Build history of the part. All positions in model axes, mm. Round coordinates to 2 decimals unless told otherwise and drop trailing zeros. Write each loop counter-clockwise with the first axis right and the second up, starting at its lowest first coordinate (ties: lowest second). Pieces come first, ordered by that corner, then holes.
Item 1: Band-saw the part on C-C, the plane z = 0. Write the cut outline in (x, y).
Item 2: Band-saw the part on A-A, the plane x = 29. Write the cut outline in (y, z), then the cut area to 3 significant figures.
Item 3: Wall check: probe 1 along X at (y, z) = (1.05, -0.5); probe 2 along X at (y, z) = (0.2, 3); probe 3 along X at (y, z) = (1.6, 0). Give the ranges that are in metal, low to high.
Item 4: Drop flat-ended pins along their axis: pin 1 Ø1.9 at (x, z) = (29, 0) entering from -Y; pin 2 Ø2 at (x, y) = (35, 3) entering from -Z; pin 3 Ø1.5 at (y, z) = (2.5, -5) entering from -X; pin 4 Ø2 at (y, z) = (4.5, 14) entering from +X. Give the stop position or say it passes through.
Item 5: Band-saw the part on D-D, the plane x = -39. Write the cut outline in (y, z), then the cut area to 3 significant figures.
Item 6: Band-saw the part on B-B, the plane y = 1.3. Count the separate pieces of the cut face and the enclosed holes in it, then the cut area to 3 significant figures.
```python
from build123d import *

# Parameters (mm, degrees)
SKETCH_1_W          = 100
SKETCH_1_H          = 38
SKETCH_1_R          = 8
SKETCH_1_R_2        = 3.5
EXTRUDE_1_DEPTH     = 5
FILLET_1_R          = 20
MM_TRANSITIONAL_1_D = 3
HOLE_WIZARD_M2_1_D  = 2.4


with BuildPart() as part:
    # 草图1 → 凸台-拉伸1 (new body)
    with BuildSketch(Plane(origin=(0, 0, 0), x_dir=(1, 0, 0), z_dir=(0, 1, 0))):
        with Locations((0, 1)):
            Rectangle(SKETCH_1_W, SKETCH_1_H)
        with Locations(Location((0, 0, 0), (0, 0, 270))):
            Circle(SKETCH_1_R, mode=Mode.SUBTRACT)
        with Locations(Location((39, 0, 0), (0, 0, 270))):
            Circle(SKETCH_1_R_2, mode=Mode.SUBTRACT)
        with Locations(Location((-39, 0, 0), (0, 0, 90))):
            Circle(SKETCH_1_R_2, mode=Mode.SUBTRACT)
    extrude(amount=EXTRUDE_1_DEPTH)

    # 圆角1
    # the kernel refuses this fillet: 20 mm, written as the material it takes off along each edge
    with BuildSketch(Plane(origin=(-50, -50, -20), x_dir=(1, 0, 0), z_dir=(0, 1, 0))) as fillet_1_piece_1:
        with BuildLine():
            CenterArc((FILLET_1_R, -FILLET_1_R), FILLET_1_R, 90, 90)
            Line((0, -FILLET_1_R), (0, 0))
            Line((0, 0), (FILLET_1_R, 0))
        make_face()
    extrude(amount=105, mode=Mode.SUBTRACT)
    with BuildSketch(Plane(origin=(-50, -50, 18), x_dir=(1, 0, 0), z_dir=(0, 1, 0)), Plane(origin=(50, -50, -20), x_dir=(-1, 0, 0), z_dir=(0, 1, 0)), Plane(origin=(50, -50, 18), x_dir=(0, 0, -1), z_dir=(0, 1, 0))) as fillet_1_piece_2:
        with BuildLine():
            CenterArc((FILLET_1_R, FILLET_1_R), FILLET_1_R, 180, 90)
            Line((0, FILLET_1_R), (0, 0))
            Line((0, 0), (FILLET_1_R, 0))
        make_face()
    extrude(amount=105, mode=Mode.SUBTRACT)

    # 大小mm Transitional 暗销孔1 (through all)
    with Locations(Plane(origin=(0, 5, 0), x_dir=(1, 0, 0), z_dir=(0, 1, 0))):
        with Locations((14, 9), (-14, 9)):
            Hole(MM_TRANSITIONAL_1_D / 2)

    # M2 间隙孔1 (through all)
    with Locations(Plane.ZX.offset(5)):
        with Locations((-10, 39), (10, 39), (0, 29)):
            hole_wizard_m2_1 = Hole(HOLE_WIZARD_M2_1_D / 2)

    # 镜向1: M2 间隙孔1 across plane
    add(hole_wizard_m2_1.mirror(Plane(origin=(0, 0, 0), x_dir=(0, 0, 1), z_dir=(1, 0, 0))), mode=Mode.SUBTRACT)


solid = part.part
```
Results:
1. outline: (-49.9, 0) - (-42.5, 0) - (-42.5, 5) - (-49.9, 5) - close; (-35.5, 0) - (-30.2, 0) - (-30.2, 5) - (-35.5, 5) - close; (-27.8, 0) - (-8, 0) - (-8, 5) - (-27.8, 5) - close; (8, 0) - (27.8, 0) - (27.8, 5) - (8, 5) - close; (30.2, 0) - (35.5, 0) - (35.5, 5) - (30.2, 5) - close; (42.5, 0) - (49.9, 0) - (49.9, 5) - (42.5, 5) - close
2. outline: (0, -20) - (5, -20) - (5, -1.2) - (0, -1.2) - close; (0, 1.2) - (5, 1.2) - (5, 18) - (0, 18) - close
2. area: 178 mm2
3. probe 1: x = -49.94 to -42.46, -35.54 to -30.09, -27.91 to -7.98, 7.98 to 27.91, 30.09 to 35.54, 42.46 to 49.94
3. probe 2: x = -49.36 to -40.8, -37.2 to -7.42, 7.42 to 37.2, 40.8 to 49.36
3. probe 3: x = -49.9 to -42.5, -35.5 to -30.2, -27.8 to -8, 8 to 27.8, 30.2 to 35.5, 42.5 to 49.9
4. pin 1: passes through
4. pin 2: stops at z = -19.6
4. pin 3: stops at x = -49.54
4. pin 4: stops at x = 43.23
5. outline: (0, -17.86) - (5, -17.86) - (5, -11.2) - (0, -11.2) - close; (0, -8.8) - (5, -8.8) - (5, -3.5) - (0, -3.5) - close; (0, 3.5) - (5, 3.5) - (5, 8.8) - (0, 8.8) - close; (0, 11.2) - (5, 11.2) - (5, 15.86) - (0, 15.86) - close
5. area: 110 mm2
6. separate pieces: 1
6. enclosed holes: 11
6. area: 3,140 mm2
